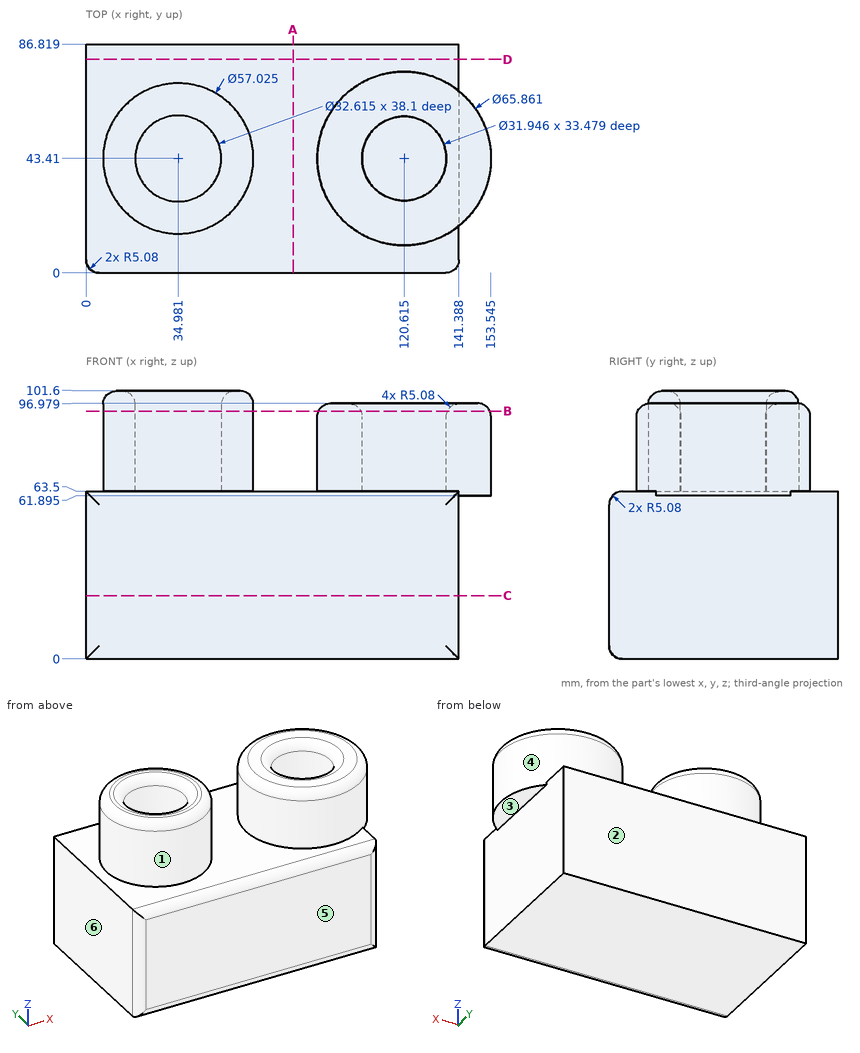
Input: dimensioned drawing with shaded views. Units: mm. Origin: part minimum x, y, z. A direction names the side the tool comes from. Round coordinates to 2 decimals unless told otherwise and drop trailing zeros. Order: outer loops, then holes, each group sorted by start corner. A loop starts at its lowest first (then second) coordinate and runs counter-clockwise, first axis right, second up.
Q1. Section D-D, the plane y = 81. Output: boundary loops of the cut face in (x, z), and give its area (3 significant figures).
Result sheet:
outline: (0, 0) - (141.39, 0) - (141.39, 63.5) - (0, 63.5) - close
area: 8,980 mm2
Q2. Section C-C, the plane z = 24. Output: boundary loops of the cut face in (x, y), and give its area (3 significant figures).
Result sheet:
outline: (0, 5.08) arc R5.08 ccw to (5.08, 0) - (136.31, 0) arc R5.08 ccw to (141.39, 5.08) - (141.39, 86.82) - (0, 86.82) - close
area: 12,300 mm2
Q3. Pin query (flat end, axial travel): pin 1 (1 mm diameter, centred on y = 55.5, z = 59, fed in from +X); pin 2 (10 mm diameter, centred on x = 31.5, y = 43.5, fed in from +Z); pin 3 (24.5 mm diameter, centred on x = 96.5, y = 36, fed in from +Z). Return the tip coordinate at first contact, or that it passes through.
Result sheet:
pin 1: stops at x = 141.39
pin 2: stops at z = 63.5
pin 3: stops at z = 96.98
Q4. Access query for the marked faces 1, 2 and 3. Directions: +Z, -Z, +X, -X, +Y, -Y. A direction counts if a zero-diameter tool reaches every point of the face in a straight line with its end or side. Return the directions, or none.
Result sheet:
face 1: +Z
face 2: +Z, -Z, +X, -X, +Y
face 3: -Z, +X, +Y, -Y
Q5. Section A-A, the plane x = 78.5. Output: boundary loops of the cut face in (y, z).
Result sheet:
outline: (0, 5.08) arc R5.08 ccw to (5.08, 0) - (86.82, 0) - (86.82, 63.5) - (5.08, 63.5) arc R5.08 ccw to (0, 58.42) - close
Q6. Material intervals for probe 1 along Z at (x, y) = (121, 19); probe 2 along Z at (x, y) = (144, 48) (1 decimal); probe 3 along X at (y, z) = (76, 37), sorted ascending.
Result sheet:
probe 1: z = 0 to 96.98
probe 2: z = 61.9 to 97
probe 3: x = 0 to 141.39
Q7. Mould query, pull axis X, two halves, no side actions, for the marked faces 4, 5 and 6. Classes: released by +X, released by -X, zero draft, split by the parting line, or undercut.
Result sheet:
face 4: undercut
face 5: zero draft
face 6: released by -X
Q8. Section B-B, the plane z = 94. Give the number of separate pieces and of enclosed holes in the cut face, and give its area (3 significant figures).
Result sheet:
separate pieces: 2
enclosed holes: 2
area: 4,180 mm2
